The drawing under review shows one solid part. Ordinate dimensions are in mm from its lowest x, y, z. Round coordinates to 2 decimals unless told otherwise and drop trailing zeros. Order: outer loops, then holes, each group sorted by start corner. A loop starts at its lowest first (then second) coordinate and runs counter-clockwise, first axis right, second up. Notation, with made-up numbers: M -38,52.25 L 1,52.25 A23 cw 1,71.25 Z; hole C 10.5,85.5 d6. An arc over 180 degrees is marked long. Answer as a JSON object with one key per item and string values.
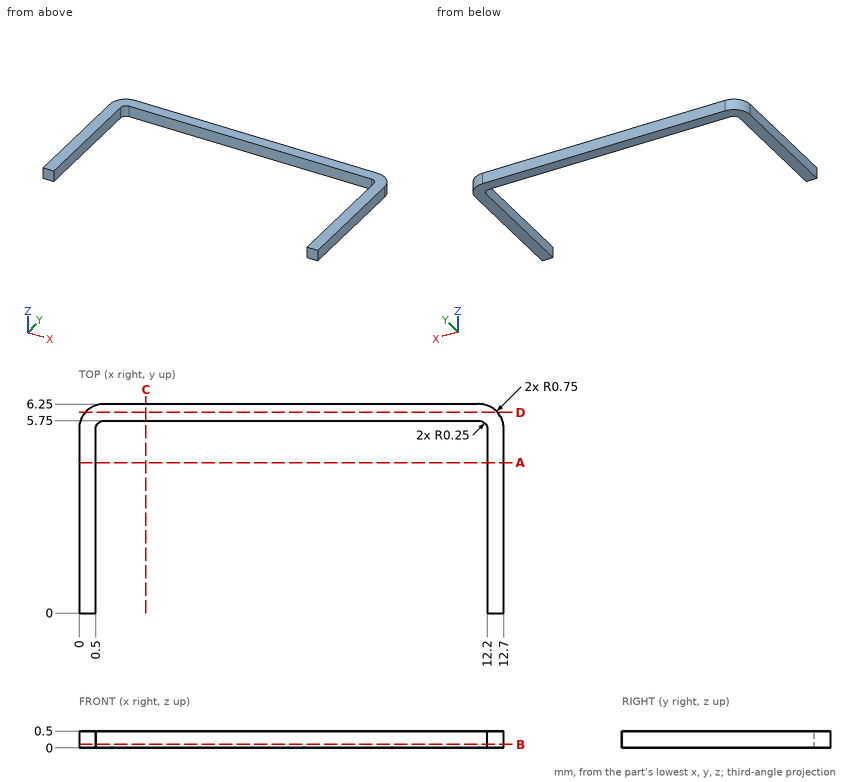
1) For L1, parallel to X at y = 5.25, z = 0.4; L2, parallel to Y at x = 9.25, z = 0.3, list the stretches that pass through material, from the lowest coordinate up.
Geometry check:
{"L1": "x = 0 to 0.5, 12.2 to 12.7", "L2": "y = 5.75 to 6.25"}
2) Add section C-C on x = 2. State the section outline as (y, z) points, and give its area (3 significant figures).
Geometry check:
{"outline": "M 5.75,0 L 6.25,0 L 6.25,0.5 L 5.75,0.5 Z", "area": "0.250 mm²"}
3) Add section D-D on y = 6. State the section outline as (x, z) points, and give its area (3 significant figures).
Geometry check:
{"outline": "M 0.19,0 L 12.51,0 L 12.51,0.5 L 0.19,0.5 Z", "area": "6.16 mm²"}
4) Add section A-A on y = 4.5. State the section outline as (x, z) points, and give its area (3 significant figures).
Geometry check:
{"outline": "M 0,0 L 0.5,0 L 0.5,0.5 L 0,0.5 Z; M 12.2,0 L 12.7,0 L 12.7,0.5 L 12.2,0.5 Z", "area": "0.500 mm²"}
5) Add section B-B on z = 0.1. State the section outline as (x, y) points, and give its area (3 significant figures).
Geometry check:
{"outline": "M 0,0 L 0.5,0 L 0.5,5.5 A0.25 cw 0.75,5.75 L 11.95,5.75 A0.25 cw 12.2,5.5 L 12.2,0 L 12.7,0 L 12.7,5.5 A0.75 ccw 11.95,6.25 L 0.75,6.25 A0.75 ccw 0,5.5 Z", "area": "11.9 mm²"}
